```python
from build123d import *

# Parameters (mm, degrees)
BOSS_EXTRUDE1_DEPTH  = 30
SHELL1_T             = -7
SKETCH2_R            = 15
CUT_EXTRUDE1_DEPTH   = 20
SKETCH3_R            = 2.805999004
CUT_EXTRUDE2_DEPTH   = 20
LPATTERN1_COUNT      = 2
LPATTERN1_PITCH      = 47
LPATTERN1_COUNT_DIR2 = 2
LPATTERN1_PITCH_DIR2 = 47
SKETCH4_W            = 38.622861656
SKETCH4_H            = 38.365375911
CUT_EXTRUDE3_DEPTH   = 20


with BuildPart() as part:
    # Sketch1 → Boss-Extrude1 (new body)
    with BuildSketch(Plane.XY):
        with BuildLine():
            Line((-48.579903717, 70.777906396), (-98.579903717, 20.777906396))
            Line((-98.579903717, 20.777906396), (-98.579903717, -49.222093604))
            Line((-98.579903717, -49.222093604), (81.420096283, -49.222093604))
            Line((81.420096283, -49.222093604), (81.420096283, 69.777906396))
            ThreePointArc((81.420096283, 69.777906396), (81.127203064, 70.485013177), (80.420096283, 70.777906396))
            Line((80.420096283, 70.777906396), (-48.579903717, 70.777906396))
        make_face()
    extrude(amount=BOSS_EXTRUDE1_DEPTH)

    # Shell1
    shell1_openings = [part.faces().sort_by_distance(p)[0] for p in [
        (-4.076298463, 8.11549528, 30),
    ]]
    offset(amount=SHELL1_T, openings=shell1_openings, kind=Kind.INTERSECTION)

    # Sketch2 → Cut-Extrude1 (cut)
    with BuildSketch(Plane.XY.offset(7)):
        with Locations((-58.579903717, -9.222093604)):
            Circle(SKETCH2_R)
    extrude(amount=-CUT_EXTRUDE1_DEPTH, mode=Mode.SUBTRACT)

    # Sketch3 → Cut-Extrude2 (cut)
    with BuildSketch(Plane.XY.offset(7)):
        with Locations((-82.079903717, 14.277906396)):
            Circle(SKETCH3_R)
    cut_extrude2 = extrude(amount=-CUT_EXTRUDE2_DEPTH, mode=Mode.SUBTRACT)

    # LPattern1: Cut-Extrude2 2 × 2
    with Locations(*[(i * LPATTERN1_PITCH, -j * LPATTERN1_PITCH_DIR2, 0) for i in range(LPATTERN1_COUNT) for j in range(LPATTERN1_COUNT_DIR2) if (i, j) != (0, 0)]):
        add(cut_extrude2, mode=Mode.SUBTRACT)

    # Sketch4 → Cut-Extrude3 (cut)
    with BuildSketch(Plane.XY.offset(7)):
        with Locations((1.108051651, 27.962073286)):
            Rectangle(SKETCH4_W, SKETCH4_H)
    extrude(amount=-CUT_EXTRUDE3_DEPTH, mode=Mode.SUBTRACT)


solid = part.part
```
Geometry: final body of the model. Coordinates: model frame, mm. A direction names the side the tool comes from. Give positions to 0.01 mm unless a question says otherwise; leave off trailing zeros. Write each loop counter-clockwise with the first axis right and the second up, starting at its lowest first coordinate (ties: lowest second). Pieces come first, ordered by that corner, then holes.
1. Section query A-A, the plane z = 24. Return loops of the section in (x, y).
2. Section query D-D, the plane x = 27.5. Return loops of the section in (y, z).
3. Pin query (flat end, axial travel): P1, Ø2, axis at y = 25.5, z = 2, coming from the -X side; P2, Ø4, axis at x = -34.5, y = 37.5, coming from the +Z side; P3, Ø1.5, axis at y = 40.5, z = 22.5, coming from the -X side. Return the tip coordinate at first contact, or that it passes through.
4. Line query: probe 1 along Y at (x, z) = (33.5, 19.75); probe 2 along X at (y, z) = (-34.5, 15.75); probe 3 along Z at (x, y) = (-69.5, 9). Output: solid intervals per line, ascending.
5. Section query C-C, the plane y = -1.5. Return loops of the section in (x, z), then the cut area to 3 significant figures.
6. Draft query along X for faces 1 (the flat face through (-10, -42.222, 18)), 2 (the flat face through (-10, -49.222, 15)), 3 (the flat face through (81.42, 9, 15)), 4 (the flat face through (-73.23, 46.13, 14.79)). Return one class per face: released by +X, released by -X, zero draft, split by the parting line, or undercut.
7. Section query B-B, the plane x = 4. Return loops of the section in (y, z), then the cut area to 3 significant figures.
8. Reachability of faces 5 (the flat face through (20.419, 28, 4)), 6 (the flat face through (-10, -2, 0)), 7 (the flat face through (15, 63.778, 18)) from +Z, -Z, +X, -X, +Y, -Y: full face, straight path, thin tool, end or side. Return the list, or none.
Computed:
1. outline: (-98.58, -49.22) - (81.42, -49.22) - (81.42, 69.78) arc R1 ccw to (80.42, 70.78) - (-48.58, 70.78) - (-98.58, 20.78) - close; hole (-91.58, -42.22) - (74.42, -42.22) - (74.42, 63.78) - (-45.68, 63.78) - (-91.58, 17.88) - close
2. outline: (-49.22, 0) - (70.78, 0) - (70.78, 30) - (63.78, 30) - (63.78, 7) - (-42.22, 7) - (-42.22, 30) - (-49.22, 30) - close
3. P1: stops at x = -94.86
3. P2: stops at z = 7
3. P3: stops at x = -79.61
4. probe 1: y = -49.22 to -42.22, 63.78 to 70.78
4. probe 2: x = -98.58 to -91.58, 74.42 to 81.42
4. probe 3: z = 0 to 7
5. outline: (-98.58, 0) - (-71.44, 0) - (-71.44, 7) - (-91.58, 7) - (-91.58, 30) - (-98.58, 30) - close; (-45.72, 0) - (81.42, 0) - (81.42, 30) - (74.42, 30) - (74.42, 7) - (-45.72, 7) - close
5. area: 1,400 mm2
6. face 1: undercut
6. face 2: zero draft
6. face 3: released by +X
6. face 4: released by -X
7. outline: (-49.22, 0) - (8.78, 0) - (8.78, 7) - (-42.22, 7) - (-42.22, 30) - (-49.22, 30) - close; (47.14, 0) - (70.78, 0) - (70.78, 30) - (63.78, 30) - (63.78, 7) - (47.14, 7) - close
7. area: 893 mm2
8. face 5: +Z, -Z
8. face 6: -Z, +X, -X, +Y, -Y
8. face 7: +Z
